Input: part model. Units: mm. Frame: model coordinates. A direction names the side the tool comes from. Give positions to 0.01 mm unless a question says otherwise; leave off trailing zeros. Write each loop counter-clockwise with the first axis right and the second up, starting at its lowest first coordinate (ties: lowest second). Pieces come first, ordered by that corner, then holes. Notation, with made-up numbers: (16.5, -16.5) - (66.5, -16.5) arc R26 ccw to (66.5, 16.5) - close; hole circle Ø4 at (81.5, -1). An arc over 180 degrees is marked (long way). Use a Markdown table: item, result. Add a question column.
1. Section query B-B, the plane x = 63.6. Return loops of the section in (y, z), plus the area to 3 significant figures.
2. Section query C-C, the plane z = -0.35. Return loops of the section in (x, y), plus the area to 3 significant figures.
3. Pin query (flat end, axial travel): pin 1 (0.7 mm diameter, centred on x = 64, y = 11.5, fed in from -Z); pin 2 (2 mm diameter, centred on x = 64, z = -0.5, fed in from +Y). Return the tip coordinate at first contact, or that it passes through.
4. Mould query, pull axis Y, two halves, no side actions, for faces 1 (the flat face through (64, 12, -0.9)), 2 (the cylindrical face through (65.794, 12.191, 0.03)), 3 (the flat face through (64, 14, 1.5)). Classes: released by +Y, released by -Y, zero draft, split by the parting line, or undercut.
5. Section query A-A, the plane y = 11.5. Return loops of the section in (x, z).
6. Set-up query: faces 4 (the cylindrical face through (63.5, 8.7, 2.2)), 5 (the flat face through (63.175, 14.7, 2.2)), 6 (the flat face through (64.025, 14.7, 2.2)). Return all of +Z, -Z, +X, -X, +Y, -Y with unobstructed straight access to the full face (end or side cutting, diameter ignored); none if empty.
7. Material intervals for probe 1 along Z at (x, y) = (62.75, 11.5); probe 2 along Y at (x, z) = (64.55, -0.95); probe 3 along Y at (x, z) = (63.7, 0.3), sorted ascending.
```python
from build123d import *

# Parameters (mm, degrees)
SKETCH055_R     = 2.3
PAD038_DEPTH    = 3
PAD039_DEPTH    = 1.5
SKETCH057_W     = 2.2
SKETCH057_H     = 2.2
POCKET010_DEPTH = 0.6
CHAMFER004_SIZE = 0.1


with BuildPart() as part:
    # Sketch055 → Pad038 (new body)
    with BuildSketch(Plane.XY):
        Circle(SKETCH055_R)
    extrude(amount=PAD038_DEPTH)

    # Sketch056 (on Face3 of Pad038) → Pad039 (join)
    with BuildSketch(Plane.XY.offset(3)):
        with BuildLine():
            Line((0.425, 2.767558), (0.425, 3.617558))
            Line((0.425, 3.617558), (-0.425, 3.617558))
            Line((-0.425, 3.617558), (-0.425, 2.767558))
            ThreePointArc((-0.425, 2.767558), (0, -2.8), (0.425, 2.767558))
        make_face()
    extrude(amount=PAD039_DEPTH)

    # Sketch057 → Pocket010 (cut)
    with BuildSketch(Plane.XY):
        Rectangle(SKETCH057_W, SKETCH057_H)
    extrude(amount=POCKET010_DEPTH, mode=Mode.SUBTRACT)

    # Chamfer004
    chamfer004_edges = [part.edges().sort_by_distance(p)[0] for p in [
        (0, 1.1, 0),
        (0, -1.1, 0),
        (1.1, 0, 0),
        (-2.3, 0, 0),
        (-1.1, 0, 0),
    ]]
    chamfer(chamfer004_edges, length=CHAMFER004_SIZE)


with BuildPart() as part_1:
    # Body016 placement: moved
    add(part.part.moved(Location((63.6, 11.5, -1.5))))


solid = part_1.part
```
Result sheet:
| question | item | result |
|---|---|---|
| 1 | outline | (8.7, 1.5) - (9.2, 1.5) - (9.2, -1.4) - (9.3, -1.5) - (10.3, -1.5) - (10.4, -1.4) - (10.4, -0.9) - (12.6, -0.9) - (12.6, -1.4) - (12.7, -1.5) - (13.7, -1.5) - (13.8, -1.4) - (13.8, 1.5) - (15.12, 1.5) - (15.12, 3) - (8.7, 3) - close |
| 1 | area | 22.1 mm² |
| 2 | outline | circle Ø4.6 at (63.6, 11.5) |
| 2 | area | 16.6 mm² |
| 3 | pin 1 | stops at z = -0.9 |
| 3 | pin 2 | stops at y = 13.8 |
| 4 | face 1 | undercut |
| 4 | face 2 | split by the parting line |
| 4 | face 3 | zero draft |
| 5 | outline | (60.8, 1.5) - (61.3, 1.5) - (61.3, -1.4) - (61.4, -1.5) - (62.4, -1.5) - (62.5, -1.4) - (62.5, -0.9) - (64.7, -0.9) - (64.7, -1.4) - (64.8, -1.5) - (65.8, -1.5) - (65.9, -1.4) - (65.9, 1.5) - (66.4, 1.5) - (66.4, 3) - (60.8, 3) - close |
| 6 | face 4 | +Z, -Z |
| 6 | face 5 | +Z, -Z, -X, +Y |
| 6 | face 6 | +Z, -Z, +X, +Y |
| 7 | probe 1 | z = -0.9 to 3 |
| 7 | probe 2 | y = 9.41 to 10.4, 12.6 to 13.59 |
| 7 | probe 3 | y = 9.2 to 13.8 |
